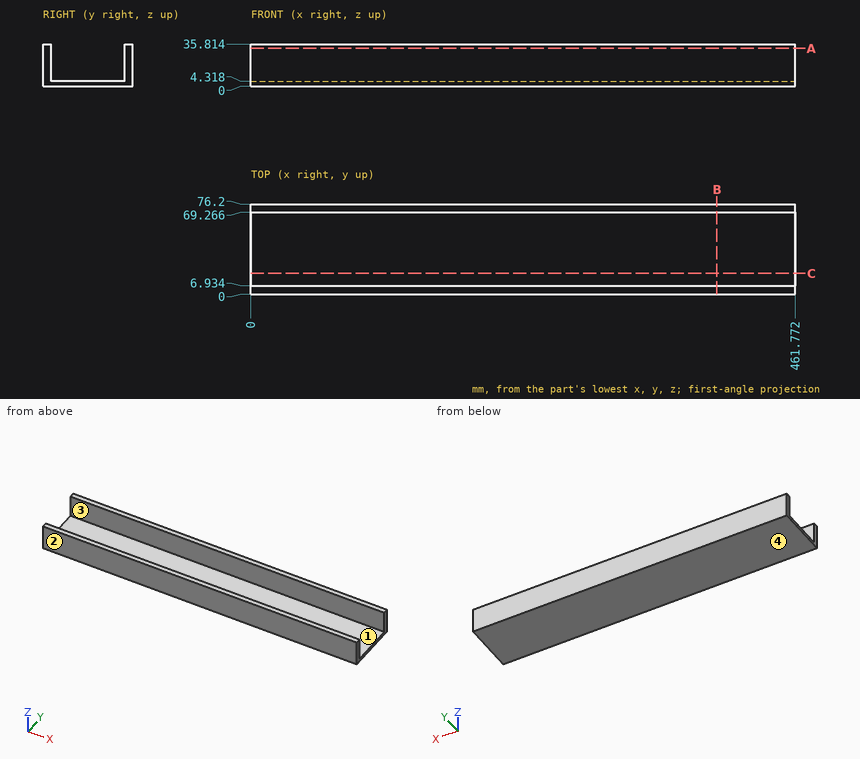
Here's the drawing with two shaded views (mm, measured from the low corner). I have some questions. Coordinates: 2 decimals unless noted, no trailing zeros. Order: outer loops, then holes, each group sorted by start corner. A loop starts at its lowest first (then second) coordinate and runs counter-clockwise, first axis right, second up.
Item 1: I need wall thicknesses on line 1 (Y direction, x = 237.5, z = 13.5); line 2 (Z direction, x = 440.5, y = 66.5). Which ranges of each line are inside material? Lowest first, please.
Result sheet:
line 1: y = 0 to 6.93, 69.27 to 76.2
line 2: z = 0 to 4.32
Item 2: If we section it at B-B on x = 395.5: List the corners of the cut face in (y, z) for me, plus the area to 3 significant figures.
Result sheet:
outline: (0, 0) - (76.2, 0) - (76.2, 35.81) - (69.27, 35.81) - (69.27, 4.32) - (6.93, 4.32) - (6.93, 35.81) - (0, 35.81) - close
area: 766 mm2
Item 3: If we mould it in two halves opening along Y, with no side actions, what happens to the marked faces 1, 2, 3 and 4? For each: +Y half, -Y half, draft (parallel to the pull), parting line (faces both ways), or undercut.
Result sheet:
face 1: undercut
face 2: -Y half
face 3: undercut
face 4: draft
Item 4: For P1, Ø3, axis at x = 201.5, y = 38.5, coming from the +Z side, with a flat end and sliding along its axis, tell me the tip position at first contact or that it passes through.
Result sheet:
P1: stops at z = 4.32
Item 5: If we section it at A-A on z = 32: List the corners of the cut face in (x, y) for me, plus the area to 3 significant figures.
Result sheet:
outline: (0, 0) - (461.77, 0) - (461.77, 6.93) - (0, 6.93) - close; (0, 69.27) - (461.77, 69.27) - (461.77, 76.2) - (0, 76.2) - close
area: 6,400 mm2
Item 6: If we section it at C-C on y = 17.5: List the corners of the cut face in (x, z) for me, plus the area to 3 significant figures.
Result sheet:
outline: (0, 0) - (461.77, 0) - (461.77, 4.32) - (0, 4.32) - close
area: 1,990 mm2
